Work out the finished part from the listing and answer in its coordinate system (mm). Coordinates: 2 decimals unless noted, no trailing zeros. Order: outer loops, then holes, each group sorted by start corner. A loop starts at its lowest first (then second) coordinate and runs counter-clockwise, first axis right, second up. Notation, with made-up numbers: (81, 20.5) - (91, 20.5) arc R31 cw to (91, 57.5) - close; hole circle Ø5 at (25, 45). An arc over 180 degrees is marked (long way). Answer as a JSON object with one key per item and string values. Group by question number.
1) Section C-C (z = 2.5) is taken. Give the vertices of the cut face in (x, y).
2) Section B-B (x = -35) is taken. Give the vertices of the cut face in (y, z), plus the area to 3 significant figures.
3) Section A-A (y = 3.6) is taken. Give the vertices of the cut face in (x, z), plus the area to 3 significant figures.
4) Section D-D (z = 5.75) is taken. Give the vertices of the cut face in (x, y).
5) This flat-tipped pin is pushed along its axis until it touches: P1, Ø1.5, axis at x = -20, z = 5, coming from the -Y side. Where does it stop, or does it pass through?
6) The mould has two halves that part along Z. Classify faces 1 (the face through (-20, 3, 10)), 2 (the face through (0, 3, 5)), 3 (the face through (-4.2, 3, 2.5)): released by +Z, released by -Z, zero draft, split by the parting line, or undercut.
7) Find the intervals of material crossed by line 1 along Z through (x, y) = (-5, 1.3); line 2 along Z through (x, y) = (-20, 3.05); line 3 along X through (y, z) = (0.35, 2), in increasing order.
Autodesk Inventor part; units mm, degrees
ref_plane "YZ Plane" through (0, 0, 0) normal (1, 0, 0) x (0, 1, 0)
ref_plane "XZ Plane" through (0, 0, 0) normal (0, 1, 0) x (-1, 0, 0)
ref_plane "XY Plane" through (0, 0, 0) normal (0, 0, 1) x (1, 0, 0)
sketch "Sketch1" plane through (0, 0, 0) normal (0, 1, 0) x (-1, 0, 0)
  line L0 (0, 10) -> (40, 10)
  line L1 (40, 10) -> (40, 0)
  line L2 (40, 0) -> (0, 0)
  line L3 (0, 0) -> (0, 10)
  circle A0 centre (5, 2.5) radius 0.8
  circle A1 centre (35, 2.5) radius 0.8
  circle A2 centre (20, 5) radius 1.25
  dimension "d0" = 1.6
  dimension "d1" = 2.5
  dimension "d2" = 5
  dimension "d3" = 5
  dimension "d4" = 30
  dimension "d5" = 10
  dimension "d8" = 2.5
  dimension "d9" = 20
  dimension "d10" = 5
extrude "Extrusion1" add sketch "Sketch1" along normal blind 6
properties part number "phone_holder_slider_insert" material "Acrylic, Clear"
Report:
{
 "1": {"outline": "(-40, 0) - (-35.8, 0) - (-35.8, 6) - (-40, 6) - close; (-34.2, 0) - (-5.8, 0) - (-5.8, 6) - (-34.2, 6) - close; (-4.2, 0) - (0, 0) - (0, 6) - (-4.2, 6) - close"},
 "2": {"outline": "(0, 0) - (6, 0) - (6, 1.7) - (0, 1.7) - close; (0, 3.3) - (6, 3.3) - (6, 10) - (0, 10) - close", "area": "50.4 mm²"},
 "3": {"outline": "(-40, 0) - (0, 0) - (0, 10) - (-40, 10) - close; hole circle Ø1.6 at (-35, 2.5); hole circle Ø2.5 at (-20, 5); hole circle Ø1.6 at (-5, 2.5)", "area": "391 mm²"},
 "4": {"outline": "(-40, 0) - (-21, 0) - (-21, 6) - (-40, 6) - close; (-19, 0) - (0, 0) - (0, 6) - (-19, 6) - close"},
 "5": {"P1": "passes through"},
 "6": {"face 1": "released by +Z", "face 2": "zero draft", "face 3": "undercut"},
 "7": {"line 1": "z = 0 to 1.7, 3.3 to 10", "line 2": "z = 0 to 3.75, 6.25 to 10", "line 3": "x = -40 to -35.62, -34.38 to -5.62, -4.38 to 0"}
}
